Input: dimensioned drawing with shaded views. Units: mm. Origin: part minimum x, y, z. A direction names the side the tool comes from. Coordinates: 2 decimals unless noted, no trailing zeros. Order: outer loops, then holes, each group sorted by start corner. A loop starts at its lowest first (then second) coordinate and runs counter-clockwise, first axis right, second up. Notation, with made-up numbers: (30, 57) - (53, 57) arc R26 ccw to (53, 89) - close; hole circle Ø11 at (29.5, -34.75). An arc over 180 degrees is marked (long way). Answer as CSV lines item,"result". Start each with the question number.
Item 1: First-contact query: pin 1 (5 mm diameter, centred on x = 21.5, z = 5, fed in from +Y); pin 2 (1 mm diameter, centred on y = 7.5, z = 3, fed in from -X); pin 3 (3 mm diameter, centred on y = 7.5, z = 3.5, fed in from +X). Flat tips, straight axial feed; report the tip coordinate or a pass-through.
Item 2: Draft query along X for the marked faces 1, 2, 3 and 4. Return one class per face: +X half, -X half, draft (parallel to the pull), parting line (faces both ways), or undercut.
Item 3: Material intervals for line 1 along Z through (x, y) = (57.5, 1.35); line 2 along Y through (x, z) = (48, 4.25); line 3 along Y through (x, z) = (10.5, 4.5), sorted ascending.
Item 4: Section C-C (y = 13.75). Output: boundary loops of the cut face in (x, z), and give its area (3 significant figures).
Item 5: Section B-B (y = 2). State how many separate pieces and enclosed holes the cut face has.
Item 6: Section D-D (z = 0.75). Output: boundary loops of the cut face in (x, y), and give its area (3 significant figures).
Item 7: Section A-A (x = 57.5). Output: boundary loops of the cut face in (y, z).
Item 8: Access query for the marked faces 5, 6 and 7. Directions: +Z, -Z, +X, -X, +Y, -Y. A direction counts if a zero-diameter tool reaches every point of the face in a straight line with its end or side. Return the directions, or none.
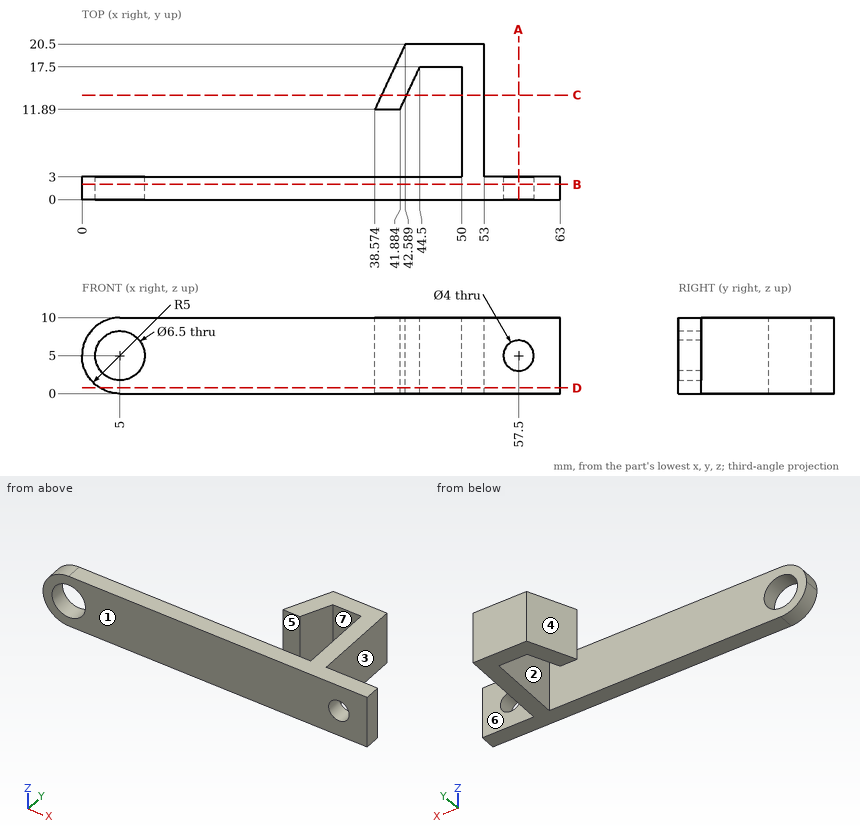
Determined:
1,pin 1,"stops at y = 3"
1,pin 2,"stops at x = 50"
1,pin 3,"stops at x = 53"
2,face 1,"draft"
2,face 2,"undercut"
2,face 3,"+X half"
2,face 4,"-X half"
3,line 1,"z = 0 to 3, 7 to 10"
3,line 2,"y = 0 to 3, 17.5 to 20.5"
3,line 3,"y = 0 to 3"
4,outline,"(39.44, 0) - (42.75, 0) - (42.75, 10) - (39.44, 10) - close; (50, 0) - (53, 0) - (53, 10) - (50, 10) - close"
4,area,"63.1 mm^2"
5,separate pieces,"1"
5,enclosed holes,"2"
6,outline,"(2.37, 0) - (63, 0) - (63, 3) - (53, 3) - (53, 20.5) - (42.59, 20.5) - (38.57, 11.89) - (41.88, 11.89) - (44.5, 17.5) - (50, 17.5) - (50, 3) - (2.37, 3) - close"
6,area,"277 mm^2"
7,outline,"(0, 0) - (3, 0) - (3, 3) - (0, 3) - close; (0, 7) - (3, 7) - (3, 10) - (0, 10) - close"
8,face 5,"+Z, -Z, -X"
8,face 6,"+Z, -Z, +X, +Y"
8,face 7,"+Z, -Z"
